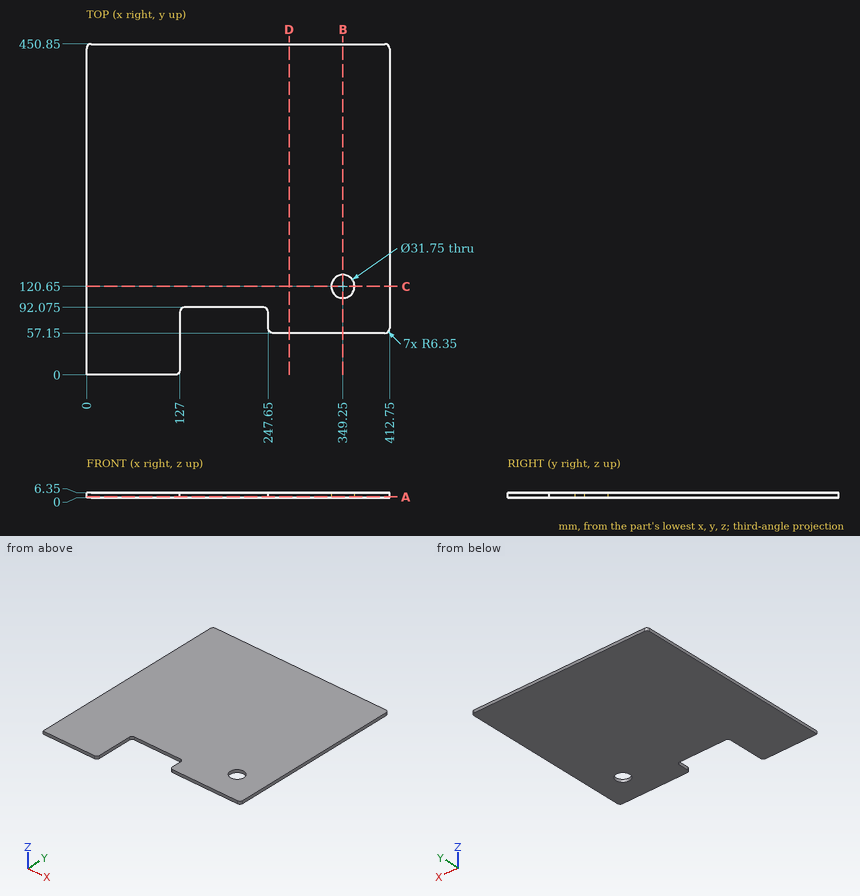
The figure shows three views and two pictorial views of one solid part (mm, origin at its lowest corner). Answer the questions. Round coordinates to 2 decimals unless told otherwise and drop trailing zeros. Order: outer loops, then holes, each group sorted by start corner. A loop starts at its lowest first (then second) coordinate and runs counter-clockwise, first axis right, second up. Notation, with made-up numbers: (29, 60) -> (37, 60) arc R31 ccw to (37, 87) -> close; hole circle Ø6 at (68.25, 33). An arc over 180 degrees is marked (long way). One line per item, written item: value.
Item 1: Straight lines are drawn through the part: L1, parallel to Y at x = 349.25, z = 5.25 (3 decimals); L2, parallel to X at y = 62.5, z = 4.5; L3, parallel to X at y = 109, z = 0.75. For each, find the intervals that lie inside material, in ascending order.
Taken from the geometry:
L1: y = 57.15 to 104.775, 136.525 to 450.85
L2: x = 0 to 127, 247.73 to 412.67
L3: x = 0 to 338.47, 360.03 to 412.75
Item 2: Find section B-B, the plane x = 349.25. Give the vertices of the cut face in (y, z) (3 decimals).
Taken from the geometry:
outline: (57.15, 0) -> (104.775, 0) -> (104.775, 6.35) -> (57.15, 6.35) -> close; (136.525, 0) -> (450.85, 0) -> (450.85, 6.35) -> (136.525, 6.35) -> close
Item 3: Find section A-A, the plane z = 1. Give the vertices of the cut face in (x, y) (3 decimals), then the cut area to 3 significant figures.
Taken from the geometry:
outline: (0, 0) -> (120.65, 0) arc R6.35 ccw to (127, 6.35) -> (127, 85.725) arc R6.35 cw to (133.35, 92.075) -> (241.3, 92.075) arc R6.35 cw to (247.65, 85.725) -> (247.65, 63.5) arc R6.35 ccw to (254, 57.15) -> (406.4, 57.15) arc R6.35 ccw to (412.75, 63.5) -> (412.75, 444.5) arc R6.35 ccw to (406.4, 450.85) -> (6.35, 450.85) arc R6.35 ccw to (0, 444.5) -> close; hole circle Ø31.75 at (349.25, 120.65)
area: 165,000 mm2
Item 4: Find section C-C, the plane y = 120.65. Give the vertices of the cut face in (x, z) (3 decimals), then the cut area to 3 significant figures.
Taken from the geometry:
outline: (0, 0) -> (333.375, 0) -> (333.375, 6.35) -> (0, 6.35) -> close; (365.125, 0) -> (412.75, 0) -> (412.75, 6.35) -> (365.125, 6.35) -> close
area: 2,420 mm2
Item 5: Find section D-D, the plane x = 276. Give the vertices of the cut face in (y, z).
Taken from the geometry:
outline: (57.15, 0) -> (450.85, 0) -> (450.85, 6.35) -> (57.15, 6.35) -> close
Item 6: Given P1, Ø3, axis at x = 347.5, z = 4, coming from the -Y side; P2, Ø1.9, axis at y = 48.5, z = 3.5, coming from the +X side; P3, Ø19, axis at x = 349.25, y = 120.65, coming from the +Z side, each flat-ended and moving along its own axis, determine where each tip first touches the part or whether it passes through.
Taken from the geometry:
P1: stops at y = 57.15
P2: stops at x = 127
P3: passes through
